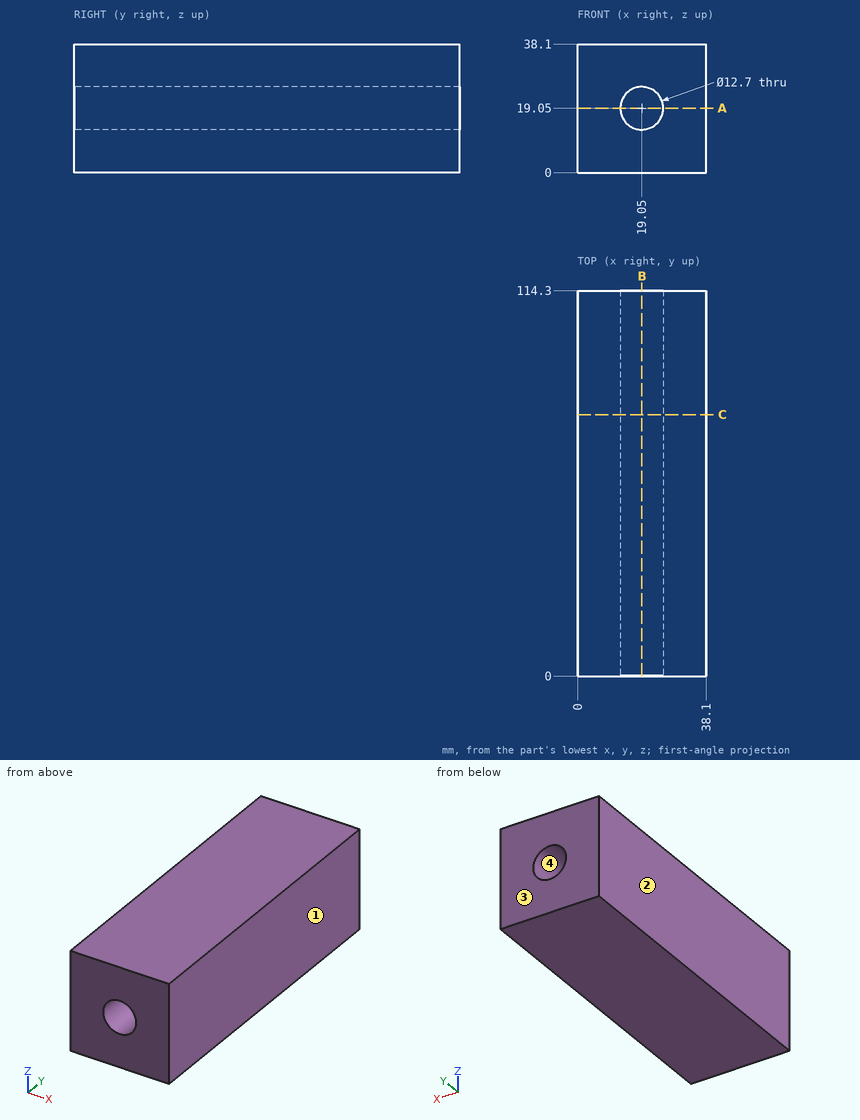
Job drawing, mm, ordinate dimensions from the low corner. One solid piece. Coordinates: 2 decimals unless noted, no trailing zeros. Order: outer loops, then holes, each group sorted by start corner. A loop starts at its lowest first (then second) coordinate and runs counter-clockwise, first axis right, second up. Notation, with made-up numbers: (0.25, 0.25) -> (49.25, 0.25) arc R21 ccw to (49.25, 39.25) -> close; hole circle Ø1 at (39.25, -17). An arc over 180 degrees is marked (long way). Put each result on its own line as item: value. Start each with the question number.
(1) Band-saw the part on C-C (y = 77.5). Give the cut face in (x, z).
(2) Band-saw the part on B-B (x = 19.05). Give the cut face in (y, z), then the cut area to 3 significant figures.
(3) Mould opens along X. For the marked faces 1, 2, 3 and 4 say: pulls with the +X half, pulls with the -X half, needs draft (parallel to the pull), parting line crosses it, or undercut.
(4) Probe line 1 along Z through (x, y) = (19.05, 31.5); line 2 along Z through (x, y) = (16, 96). List the from-to ranges inside material, lowest first. Write a range as [from, to].
(5) Band-saw the part on A-A (z = 19.05). Give the cut face in (x, y).
Determined:
1. outline: (0, 0) -> (38.1, 0) -> (38.1, 38.1) -> (0, 38.1) -> close; hole circle Ø12.7 at (19.05, 19.05)
2. outline: (0, 0) -> (114.3, 0) -> (114.3, 12.7) -> (0, 12.7) -> close; (0, 25.4) -> (114.3, 25.4) -> (114.3, 38.1) -> (0, 38.1) -> close
2. area: 2,900 mm²
3. face 1: pulls with the +X half
3. face 2: pulls with the -X half
3. face 3: needs draft
3. face 4: undercut
4. line 1: z = [0, 12.7], [25.4, 38.1]
4. line 2: z = [0, 13.48], [24.62, 38.1]
5. outline: (0, 0) -> (12.7, 0) -> (12.7, 114.3) -> (0, 114.3) -> close; (25.4, 0) -> (38.1, 0) -> (38.1, 114.3) -> (25.4, 114.3) -> close
